Check sheet for the modelled part. Datum: model origin and axes. Units: mm. A direction names the side the tool comes from. Round coordinates to 2 decimals unless told otherwise and drop trailing zeros. Order: outer loops, then holes, each group sorted by start corner. A loop starts at its lowest first (then second) coordinate and runs counter-clockwise, first axis right, second up.
Q1. Cross-section at B-B on y = -10. Record the cut outline in (x, z).
Q2. Cross-section at C-C on z = 32.5. Record the cut outline in (x, y), then the cut area to 3 significant figures.
Q3. Cross-section at A-A on x = -23. Record the cut outline in (y, z).
Q4. Mould release check, pull along Z, two halves, no side actions. Record for faces 3 (the flat face through (0, -10, 36)), 4 (the flat face through (0, 0, 18)), 5 (the flat face through (0, -16, 0)): +Z half, -Z half, draft (parallel to the pull), parting line (faces both ways), or undercut.
Q5. Scan lines: probe 1 along X at (y, z) = (-10, 13); probe 2 along Y at (x, z) = (23, 13); probe 3 along Y at (x, z) = (-23, 29.5). Record each from-to range of solid material in increasing order.
Q6. Cross-section at D-D on x = 17. Record the cut outline in (y, z).
Q7. Depth check by flat-ended pin: P1, Ø11, axis at x = 23, y = -10, coming from the +Z side; P2, Ø12, axis at x = 0, z = 30, coming from the -Y side; P3, Ø4, axis at x = -0.5, y = -24, coming from the +Z side; P4, Ø0.8, axis at x = -12.5, y = -32.5, coming from the +Z side. Enter the tip coordinate at first touch or a pass-through.
Q8. Set-up check for faces 1 (the flat face through (30, -13, 14)), 2 (the flat face through (0, -20, 31)): record each of +Z, -Z, +X, -X, +Y, -Y from which the full face is reachable in a straight line by a thin tool's end or side.
from build123d import *

# Parameters (mm, degrees)
SKETCH_W     = 60
SKETCH_H     = 36
PAD_DEPTH    = 20
SKETCH001_R  = 3.5
POCKET_DEPTH = 36.001
SKETCH004_W  = 60
SKETCH004_H  = 15
PAD003_DEPTH = 13
PAD004_DEPTH = 60


with BuildPart() as part:
    # Sketch → Pad (new body)
    with BuildSketch(Plane.XZ):
        with Locations((0, 18)):
            Rectangle(SKETCH_W, SKETCH_H)
    extrude(amount=PAD_DEPTH)

    # Sketch001 (on Face3 of Pad) → Pocket (cut, through all)
    with BuildSketch(Plane(origin=(0, 0, 36), x_dir=(-1, 0, 0), z_dir=(0, 0, 1))):
        with Locations((-23, 10)):
            Circle(SKETCH001_R)
        with Locations((23, 10)):
            Circle(SKETCH001_R)
    extrude(amount=-POCKET_DEPTH, mode=Mode.SUBTRACT)

    # Sketch004 → Pad003 (join)
    with BuildSketch(Plane.XZ.offset(20)):
        with Locations((0, 7.5)):
            Rectangle(SKETCH004_W, SKETCH004_H)
    extrude(amount=PAD003_DEPTH)

    # Sketch005 (on Face2 of Pad003) → Pad004 (join)
    with BuildSketch(Plane(origin=(-30, 0, 0), x_dir=(0, 0, -1), z_dir=(-1, 0, 0))):
        with BuildLine():
            Line((-25, 20), (-15, 20))
            Line((-15, 20), (-15, 32))
            ThreePointArc((-25, 20), (-18.170827, 24.475689), (-15, 32))
        make_face()
    extrude(amount=-PAD004_DEPTH)


solid = part.part
Results found:
1. outline: (-30, 0) - (-26.5, 0) - (-26.5, 36) - (-30, 36) - close; (-19.5, 0) - (19.5, 0) - (19.5, 36) - (-19.5, 36) - close; (26.5, 0) - (30, 0) - (30, 36) - (26.5, 36) - close
2. outline: (-30, -20) - (30, -20) - (30, 0) - (-30, 0) - close; hole circle Ø7 at (-23, -10); hole circle Ø7 at (23, -10)
2. area: 1,120 mm2
3. outline: (-33, 0) - (-13.5, 0) - (-13.5, 36) - (-20, 36) - (-20, 25) arc R14 cw to (-32, 15) - (-33, 15) - close; (-6.5, 0) - (0, 0) - (0, 36) - (-6.5, 36) - close
4. face 3: +Z half
4. face 4: draft
4. face 5: -Z half
5. probe 1: x = -30 to -26.5, -19.5 to 19.5, 26.5 to 30
5. probe 2: y = -33 to -13.5, -6.5 to 0
5. probe 3: y = -20 to -13.5, -6.5 to 0
6. outline: (-33, 0) - (0, 0) - (0, 36) - (-20, 36) - (-20, 25) arc R14 cw to (-32, 15) - (-33, 15) - close
7. P1: stops at z = 36
7. P2: stops at y = -20.33
7. P3: stops at z = 20.85
7. P4: stops at z = 15
8. face 1: +Z, -Z, +X, +Y, -Y
8. face 2: +Z, +X, -X, -Y
